Could you check a few things on this model? Use its own coordinates, in mm. A direction names the side the tool comes from. Coordinates: 2 decimals unless noted, no trailing zeros. Write each loop counter-clockwise with the first axis right and the second up, starting at its lowest first coordinate (ties: lowest second). Pieces come first, ordered by that corner, then holes. Notation, with made-up numbers: (81.5, -39.5) - (124.5, -39.5) arc R22 ccw to (124.5, -23.5) - close; hole circle Ø11 at (53.25, 68). An arc over 180 degrees is marked (long way). Write item = value, one per line. Start each with the question number.
```python
from build123d import *

# Parameters (mm, degrees)
SKETCH1_R           = 25.4
SKETCH1_R_2         = 2.65
BOSS_EXTRUDE1_DEPTH = 4
SKETCH2_R           = 2.6
BOSS_EXTRUDE2_DEPTH = 8
CUT_EXTRUDE2_START  = -2
SKETCH3_R           = 9.525
CUT_EXTRUDE2_DEPTH  = 10


with BuildPart() as part:
    # Sketch1 → Boss-Extrude1 (new body)
    with BuildSketch(Plane.XY):
        with Locations((674.616590385, -1255.036738659)):
            Circle(SKETCH1_R)
        with Locations((674.616590385, -1255.036738659)):
            Circle(SKETCH1_R_2, mode=Mode.SUBTRACT)
        with BuildLine():
            Line((661.61077501, -1252.128812685), (655.122370806, -1252.128812685))
            ThreePointArc((655.122370806, -1252.128812685), (674.616590385, -1235.326826673), (694.110809965, -1252.128812685))
            Line((694.110809965, -1252.128812685), (687.622405761, -1252.128812685))
            ThreePointArc((687.622405761, -1252.128812685), (674.616590385, -1241.709801012), (661.61077501, -1252.128812685))
        make_face(mode=Mode.SUBTRACT)
        with BuildLine():
            Line((661.61077501, -1257.944664633), (655.122370806, -1257.944664633))
            ThreePointArc((655.122370806, -1257.944664633), (674.616590385, -1274.746650645), (694.110809965, -1257.944664633))
            Line((694.110809965, -1257.944664633), (687.622405761, -1257.944664633))
            ThreePointArc((687.622405761, -1257.944664633), (674.616590385, -1268.363676307), (661.61077501, -1257.944664633))
        make_face(mode=Mode.SUBTRACT)
    extrude(amount=BOSS_EXTRUDE1_DEPTH)

    # Sketch2 → Boss-Extrude2 (add)
    with BuildSketch(Plane.XY.offset(4)):
        with Locations((652.866731087, -1255.036738659)):
            Circle(SKETCH2_R)
    extrude(amount=BOSS_EXTRUDE2_DEPTH)

    # Sketch3 → Cut-Extrude2 (cut)
    with BuildSketch(Plane(origin=(0, 0, 0), x_dir=(-1, 0, 0), z_dir=(0, 0, -1)).offset(CUT_EXTRUDE2_START)):
        with Locations((-674.616590385, -1255.036738659)):
            Circle(SKETCH3_R)
    extrude(amount=-CUT_EXTRUDE2_DEPTH, mode=Mode.SUBTRACT)


solid = part.part
```
1) Which directions (+Z, -Z, +X, -X, +Y, -Y) give clear straight access to the entire face, cutting with the end or side of a thin tool? Please do faces 1 (the cylindrical face through (652.303, -1257.575, 7.944)), 2 (the flat face through (653, -1255, 12)), 3 (the cylindrical face through (674.224, -1274.743, 1.972)).
2) Suppose I cut it at C-C on y = -1265.5. Please give me the cut outline in (x, z).
3) For P1, Ø3, axis at x = 690.5, z = 2, coming from the -Y side; P2, Ø1.2, axis at x = 657, z = 1.5, coming from the +Y side; P3, Ø21, axis at x = 673, y = -1252, coming from the +Z side, each with a flat end and sliding along its axis, tell me the tip position at first contact or that it passes through.
4) Suppose I cut it at A-A on x = 669.5. Please give me the cut outline in (y, z).
5) Thinking about a two-plate mould opening in X: for faces 4 (the flat face through (658, -1252.129, 2)), 5 (the flat face through (680, -1255, 0)), 6 (the cylindrical face through (671.31, -1229.853, 1.972)), which applies, +X half, -X half, draft (parallel to the pull), parting line (faces both ways), or undercut?
6) If I drill on probe 1 along X at (y, z) = (-1262, 1.5); probe 2 along Y at (x, z) = (657, 0.75); probe 3 along Y at (x, z) = (687, 1.25), over which ranges is the centre line in solid material (lowest first)? Write a range as [from, to].
7) Suppose I cut it at D-D on x = 675. Please give me the cut outline in (y, z).
8) Suppose I cut it at B-B on y = -1238. Please give me the cut outline in (x, z).
Reply:
q1.face_1 = +Z
q1.face_2 = +Z, +X, -X, +Y, -Y
q1.face_3 = +Z, -Z
q2.outline = (651.47, 0) - (657.91, 0) - (657.91, 4) - (651.47, 4) - close; (666.36, 0) - (682.87, 0) - (682.87, 4) - (666.36, 4) - close; (691.32, 0) - (697.76, 0) - (697.76, 4) - (691.32, 4) - close
q3.P1 = -1275.97
q3.P2 = -1236.18
q3.P3 = 4
q4.outline = (-1279.92, 0) - (-1274.07, 0) - (-1274.07, 4) - (-1279.92, 4) - close; (-1267.34, 0) - (-1242.73, 0) - (-1242.73, 4) - (-1247, 4) - (-1247, 2) - (-1263.07, 2) - (-1263.07, 4) - (-1267.34, 4) - close; (-1236, 0) - (-1230.16, 0) - (-1230.16, 4) - (-1236, 4) - close
q5.face_4 = undercut
q5.face_5 = draft
q5.face_6 = parting line
q6.probe_1 = [650.19, 656.18], [663.25, 685.98], [693.06, 699.04]
q6.probe_2 = [-1273.33, -1263.88], [-1257.94, -1252.13], [-1246.2, -1236.74]
q6.probe_3 = [-1277.21, -1270.37], [-1259.96, -1250.11], [-1239.7, -1232.86]
q7.outline = (-1280.43, 0) - (-1274.74, 0) - (-1274.74, 4) - (-1280.43, 4) - close; (-1268.36, 0) - (-1257.66, 0) - (-1257.66, 2) - (-1264.55, 2) - (-1264.55, 4) - (-1268.36, 4) - close; (-1252.41, 0) - (-1241.72, 0) - (-1241.72, 4) - (-1245.52, 4) - (-1245.52, 2) - (-1252.41, 2) - close; (-1235.33, 0) - (-1229.64, 0) - (-1229.64, 4) - (-1235.33, 4) - close
q8.outline = (655.78, 0) - (664.71, 0) - (664.71, 4) - (655.78, 4) - close; (684.53, 0) - (693.46, 0) - (693.46, 4) - (684.53, 4) - close
